The listing builds one solid part. Answer for the finished solid, in the listing's coordinates (mm). Give positions to 0.01 mm unless a question says otherwise; leave off trailing zeros. Write each loop counter-clockwise with the first axis right and the second up, starting at its lowest first coordinate (ties: lowest second). Pieces come first, ordered by that corner, then holes.
Autodesk Inventor part; units mm, degrees
ref_plane "YZ Plane" through (0, 0, 0) normal (1, 0, 0) x (0, 1, 0)
ref_plane "XY Plane" through (0, 0, 0) normal (0, 0, 1) x (1, 0, 0)
sketch "Sketch1" plane through (0, 0, 0) normal (0, 1, 0) x (-1, 0, 0)
  circle A0 centre (0, 0) radius 4.5
  circle A1 centre (0, 0) radius 3
  dimension "d0" = 9
  dimension "d1" = 6
extrude "Extrusion1" add sketch "Sketch1" along normal blind 260
ref_plane "Work Plane1" through (0, 130, 0) normal (0, 1, 0) x (-1, 0, 0)
sketch "Sketch2" plane through (0, 260, 0) normal (0, 1, 0) x (1, 0, 0)
  circle A0 centre (0, 3.75) radius 0.5
  point P0 (0, 0)
  dimension "d4" = 1
  dimension "d5" = 3.75
extrude "Extrusion2" cut sketch "Sketch2" against normal through all
mirror "Mirror1" about plane through (0, 0, 0) normal (0, 0, 1) of "Extrusion2"
properties part number "extended_shaft"
Item 1: A cutting plane is placed at B-B, the plane y = 82. Give the vertices of the cut face in (x, z).
Conclusion:
outline: circle Ø9 at (0, 0); hole circle Ø6 at (0, 0); hole circle Ø1 at (0, -3.75); hole circle Ø1 at (0, 3.75)
Item 2: A cutting plane is placed at A-A, the plane z = 0. Give the vertices of the cut face in (x, y).
Conclusion:
outline: (-4.5, 0) - (-3, 0) - (-3, 260) - (-4.5, 260) - close; (3, 0) - (4.5, 0) - (4.5, 260) - (3, 260) - close
Item 3: Determine the mould class of faces 1 (the face through (-1, 260, -3)), 2 (the face through (3, 128, 0)), 3 (the face through (0.59, 128.18, -4.46)) for opening direction Z: pulls with the +Z half, pulls with the -Z half, needs draft (parallel to the pull), parting line crosses it, or undercut.
Conclusion:
face 1: needs draft
face 2: undercut
face 3: parting line crosses it
Item 4: Each of these flat-tipped pins is pushed along its axis until it touches: P1, Ø3, axis at x = -2.5, y = 105, coming from the +Z side; P2, Ø1, axis at x = -1.5, z = 1.5, coming from the +Y side; P3, Ø1, axis at x = -3, y = 59.5, coming from the -Z side; P4, Ø2, axis at y = 114, z = -3.5, coming from the +X side. Where does it stop, or does it pass through?
Conclusion:
P1: stops at z = 4.39
P2: passes through
P3: stops at z = -3.74
P4: stops at x = 3.74
Item 5: Consider probe 1 along Z at (x, y) = (0, 111); probe 2 along X at (y, z) = (211.5, -0.75); probe 3 along X at (y, z) = (116.5, -2). Determine where each line is inside the solid, lowest interval first.
Conclusion:
probe 1: z = -4.5 to -4.25, -3.25 to -3, 3 to 3.25, 4.25 to 4.5
probe 2: x = -4.44 to -2.9, 2.9 to 4.44
probe 3: x = -4.03 to -2.24, 2.24 to 4.03
